Geometry check sheet. Reference: the model listing, model coordinates, mm. A direction names the side the tool comes from. Give positions to 0.01 mm unless a question says otherwise; leave off trailing zeros. Write each loop counter-clockwise with the first axis right and the second up, starting at its lowest first coordinate (ties: lowest second). Pieces come first, ordered by that corner, then holes. Notation, with made-up numbers: (75, -25.5) - (129, -25.5) arc R18 cw to (129, 8.5) - close; hole circle Ø1 at (-35, -26.75). An arc over 180 degrees is marked (long way). One line per question, with ' | ' between items. Start each with the question number.
Q1. Set-up check for faces 1 (the face through (93.97, 13, -1)), 2 (the face through (-90.92, 13.09, -53.42)), 3 (the face through (-59.17, 5.49, 25.97)), 4 (the face through (-90.485, 10.719, 53.148)): record each of +Z, -Z, +X, -X, +Y, -Y from which the full face is reachable in a straight line by a thin tool's end or side.
Q2. Section check B-B on x = 70. Record the boundary of the cut face in (y, z), and give its area (3 significant figures).
Q3. Release check for a two-part mould opening along X. For faces 5 (the face through (87.9, 9.93, 50.62)), 6 (the face through (59.17, 5.49, 25.75)), 7 (the face through (93.97, 8, -1)), 8 (the face through (-90.92, 7.58, -53.42)) record: +X half, -X half, draft (parallel to the pull), parting line (faces both ways), or undercut.
Q4. Section check C-C on z = -9. Record the boundary of the cut face in (x, y), and give its area (3 significant figures).
Q5. Thickness scan on L1, parallel to X at y = 11, z = 4.5; L2, parallel to X at y = 8, z = -34.5; L3, parallel to Z at x = 39, y = 7. Record the ranges inside material, lowest first. Write a range as [from, to].
Q6. Gauge pin test, flat ends, axial feed: P1, Ø11, axis at x = 23, z = -28, coming from the +Y side; P2, Ø4, axis at y = 14, z = -2, coming from the +X side; P3, Ø3, axis at x = 53.5, z = 7.5, coming from the +Y side; P4, Ø11, axis at x = 54.5, y = 8, coming from the -Z side. Record the tip position at first contact, or that the pin passes through.
Q7. Section check A-A on y = 18.5. Record the boundary of the cut face in (x, z), and give its area (3 significant figures).
```python
from build123d import *

# Parameters (mm, degrees)
EXTRUDE_1_DEPTH     = 5
EXTRUDE_2_DEPTH     = 10
SKETCH_6_W          = 9.821902293
SKETCH_6_H          = 0.385172639
CUT_EXTRUDE_2_DEPTH = 0.2
SKETCH_7_W          = 24
SKETCH_7_H          = 1
EXTRUDE_6_DEPTH     = 25.5
CUT_EXTRUDE_3_DEPTH = 1
CUT_EXTRUDE_6_DEPTH = 117.5
EXTRUDE_7_DEPTH     = 1
CHAMFER_3_SIZE      = 1


with BuildPart() as part:
    # 草图1 → 凸台-拉伸1 (new body)
    with BuildSketch(Plane(origin=(0, 0, 0), x_dir=(1, 0, 0), z_dir=(0, 1, 0))):
        Polygon((-100, 54.16), (-92.36, 61.8), (92.36, 61.8), (100, 54.16), (100, -54.16), (92.36, -61.8), (-92.36, -61.8), (-100, -54.16), align=None)
    extrude(amount=EXTRUDE_1_DEPTH)

    # 草图2 → 凸台-拉伸2 (add)
    with BuildSketch(Plane(origin=(0, 5, 0), x_dir=(1, 0, 0), z_dir=(0, 1, 0))):
        Polygon((-93.97, 50.37), (-87.79, 56.55), (87.79, 56.55), (93.97, 50.37), (93.97, -50.37), (87.79, -56.55), (-87.79, -56.55), (-93.97, -50.37), align=None)
        Polygon((-92.97, -45.55), (-82.97, -55.55), (82.97, -55.55), (92.97, -45.55), (92.97, 45.55), (82.97, 55.55), (-82.97, 55.55), (-92.97, 45.55), align=None, mode=Mode.SUBTRACT)
    extrude(amount=EXTRUDE_2_DEPTH)

    # 草图6 → 切除-拉伸2 (cut)
    with BuildSketch(Plane(origin=(72.17, 0, 72.17), x_dir=(0.7071067811865479, 0, -0.7071067811865471), z_dir=(0.7071067811865471, 0, 0.7071067811865479))):
        with Locations((26.350211631, 10.419075461)):
            Rectangle(SKETCH_6_W, SKETCH_6_H)
    extrude(amount=-CUT_EXTRUDE_2_DEPTH, mode=Mode.SUBTRACT)

    # 草图7 → 凸台-拉伸6 (add)
    with BuildSketch(Plane(origin=(0, 5, 0), x_dir=(1, 0, 0), z_dir=(0, 1, 0))):
        with Locations((0, 55.05)):
            Rectangle(SKETCH_7_W, SKETCH_7_H)
        with Locations((0, 56.05)):
            Rectangle(SKETCH_7_W, SKETCH_7_H)
        with Locations((0, -55.05)):
            Rectangle(SKETCH_7_W, SKETCH_7_H)
        with Locations((0, -56.05)):
            Rectangle(SKETCH_7_W, SKETCH_7_H)
    extrude(amount=EXTRUDE_6_DEPTH)

    # 草图5 → 切除-拉伸3 (cut)
    with BuildSketch(Plane(origin=(0, 10.226489141, 0), x_dir=(1, 0, 0), z_dir=(0, 1, 0))):
        Polygon((-87.79, -56.55), (87.79, -56.55), (93.97, -50.37), (93.97, 50.37), (87.79, 56.55), (-87.79, 56.55), (-93.97, 50.37), (-93.97, -50.37), align=None)
        Polygon((87.582893219, 56.05), (93.47, 50.162893219), (93.47, -50.162893219), (87.582893219, -56.05), (-87.582893219, -56.05), (-93.47, -50.162893219), (-93.47, 50.162893219), (-87.582893219, 56.05), align=None, mode=Mode.SUBTRACT)
    extrude(amount=CUT_EXTRUDE_3_DEPTH, mode=Mode.SUBTRACT)

    # 草图13 → 切除-拉伸6 (cut)
    with BuildSketch(Plane.XY.offset(56.55)):
        Polygon((0, 24), (7.5, 24), (7.5, 26), (-7.5, 26), (-7.5, 24), align=None)
    extrude(amount=-CUT_EXTRUDE_6_DEPTH, mode=Mode.SUBTRACT)

    # 草图17 → 凸台-拉伸7 (add)
    with BuildSketch(Plane(origin=(0, 5, 0), x_dir=(1, 0, 0), z_dir=(0, 1, 0))):
        with BuildLine():
            Line((-54.17, -20.86418044), (54.17, -20.86418044))
            ThreePointArc((54.17, -20.86418044), (59.17, -25.86418044), (54.17, -30.86418044))
            Line((54.17, -30.86418044), (-54.17, -30.86418044))
            ThreePointArc((-54.17, -30.86418044), (-59.17, -25.86418044), (-54.17, -20.86418044))
        make_face()
        with BuildLine():
            Line((-54.17, 20.86418044), (54.17, 20.86418044))
            ThreePointArc((54.17, 20.86418044), (59.17, 25.86418044), (54.17, 30.86418044))
            Line((54.17, 30.86418044), (-54.17, 30.86418044))
            ThreePointArc((-54.17, 30.86418044), (-59.17, 25.86418044), (-54.17, 20.86418044))
        make_face()
    extrude(amount=EXTRUDE_7_DEPTH)

    # 倒角3
    chamfer_3_edges = [part.edges().sort_by_distance(p)[0] for p in [
        (96.18, 0, 57.98),
        (0, 0, 61.8),
        (-96.18, 0, 57.98),
        (-100, 0, 0),
        (-96.18, 0, -57.98),
        (0, 0, -61.8),
        (96.18, 0, -57.98),
        (100, 0, 0),
    ]]
    chamfer(chamfer_3_edges, length=CHAMFER_3_SIZE)


solid = part.part
```
Working result:
1) face 1: +Z, -Z, +X, +Y | face 2: -Z, -X, +Y | face 3: +Y | face 4: +Z, -X
2) outline: (0, -60.8) - (1, -61.8) - (5, -61.8) - (5, -56.55) - (10.23, -56.55) - (10.23, -56.05) - (11.23, -56.05) - (11.23, -56.55) - (15, -56.55) - (15, -55.55) - (5, -55.55) - (5, 55.55) - (15, 55.55) - (15, 56.55) - (11.23, 56.55) - (11.23, 56.05) - (10.23, 56.05) - (10.23, 56.55) - (5, 56.55) - (5, 61.8) - (1, 61.8) - (0, 60.8) - close | area: 636 mm2
3) face 5: undercut | face 6: undercut | face 7: +X half | face 8: -X half
4) outline: (-100, 1) - (-99, 0) - (99, 0) - (100, 1) - (100, 5) - (93.97, 5) - (93.97, 10.23) - (93.47, 10.23) - (93.47, 11.23) - (93.97, 11.23) - (93.97, 15) - (92.97, 15) - (92.97, 5) - (-92.97, 5) - (-92.97, 15) - (-93.97, 15) - (-93.97, 11.23) - (-93.47, 11.23) - (-93.47, 10.23) - (-93.97, 10.23) - (-93.97, 5) - (-100, 5) - close | area: 1,020 mm2
5) L1: x = [-93.47, -92.97], [92.97, 93.47] | L2: x = [-93.97, -92.97], [92.97, 93.97] | L3: z = [-56.55, -55.55], [55.55, 56.55]
6) P1: stops at y = 6 | P2: stops at x = 93.97 | P3: stops at y = 5 | P4: stops at z = -61.8
7) outline: (-12, -56.55) - (12, -56.55) - (12, -54.55) - (-12, -54.55) - close; (-12, 54.55) - (12, 54.55) - (12, 56.55) - (-12, 56.55) - close | area: 96.0 mm2
